Solid Edge part; units mm, degrees
sketch "Sketch1" plane through (0, 0, 0) normal (0, -1, 0) x (1, 0, 0)
  line L0 (-17.399, 15.748) -> (-17.399, -15.748)
  arc A0 (-17.399, -15.748) -> (-15.748, -17.399) centre (-15.748, -15.748) ccw
  line L1 (-15.748, -17.399) -> (15.748, -17.399)
  arc A1 (15.748, -17.399) -> (17.399, -15.748) centre (15.748, -15.748) ccw
  line L2 (17.399, -15.748) -> (17.399, 15.748)
  arc A2 (17.399, 15.748) -> (15.748, 17.399) centre (15.748, 15.748) ccw
  line L3 (15.748, 17.399) -> (-15.748, 17.399)
  arc A3 (-15.748, 17.399) -> (-17.399, 15.748) centre (-15.748, 15.748) ccw
  arc A4 (-19.05, -15.748) -> (-15.748, -19.05) centre (-15.748, -15.748) ccw
  line L4 (-15.748, -19.05) -> (15.748, -19.05)
  arc A5 (15.748, -19.05) -> (19.05, -15.748) centre (15.748, -15.748) ccw
  line L5 (19.05, -15.748) -> (19.05, 15.748)
  arc A6 (19.05, 15.748) -> (15.748, 19.05) centre (15.748, 15.748) ccw
  line L6 (15.748, 19.05) -> (-15.748, 19.05)
  arc A7 (-15.748, 19.05) -> (-19.05, 15.748) centre (-15.748, 15.748) ccw
  line L7 (-19.05, 15.748) -> (-19.05, -15.748)
extrude "Protrusion1" add sketch "Sketch1" against normal blind 44.45
properties material "Steel"
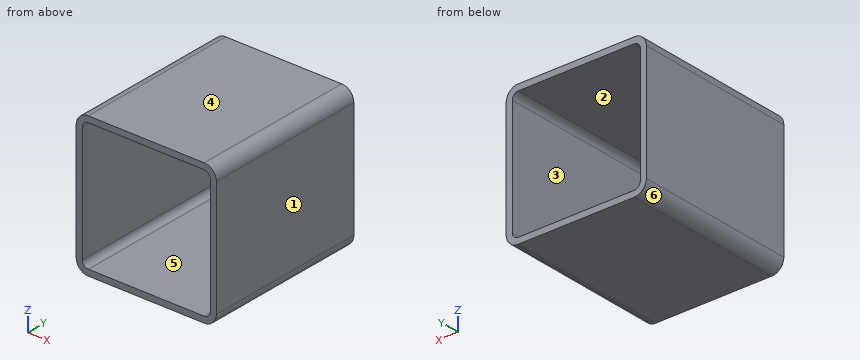
Verification items for the finished model (mm, model axes). Face numbers are marked on the shaded views. A direction names the side the tool comes from. Give positions to 0.01 mm unless a question says otherwise; leave off trailing zeros. Write each loop counter-clockwise with the first axis right and the second up, starting at its lowest first coordinate (ties: lowest second). Pieces come first, ordered by that corner, then holes. Notation, with made-up numbers: M -20,35 L 17,35 A17 cw 17,63 Z; hole C 54.5,47.25 d2. An arc over 180 degrees is marked long. Write item = value, one per line.
(1) Sectioned sample at B-B (x = -1). Record the cut outline in (y, z), then the cut area to 3 significant figures.
Found:
outline = M 0,-19.05 L 44.45,-19.05 L 44.45,-17.4 L 0,-17.4 Z; M 0,17.4 L 44.45,17.4 L 44.45,19.05 L 0,19.05 Z
area = 147 mm2
(2) Access from +Z, -Z, +X, -X, +Y, -Y to the whole of each face (thin tool, end or side, straight path). Record for the marked faces 5 and 6.
Found:
face_5 = +Y, -Y
face_6 = -Z, -X, +Y, -Y
(3) Material ranges on line 1 (X direction, y = 40, z = -5.5); line 2 (X direction, y = 3, z = 17.5), recorded low to high.
Found:
line_1 = -19.05 to -17.4, 17.4 to 19.05
line_2 = -18.55 to 18.55
(4) Draft check along Z on the marked faces 1, 2, 3 and 4. Enter one of: released by +Z, released by -Z, zero draft, split by the parting line, or undercut.
Found:
face_1 = zero draft
face_2 = undercut
face_3 = undercut
face_4 = released by +Z
(5) Sectioned sample at A-A (z = 2). Record the cut outline in (x, y).
Found:
outline = M -19.05,0 L -17.4,0 L -17.4,44.45 L -19.05,44.45 Z; M 17.4,0 L 19.05,0 L 19.05,44.45 L 17.4,44.45 Z
(6) Sectioned sample at C-C (y = 37). Record the cut outline in (x, z).
Found:
outline = M -19.05,-15.75 A3.3 ccw -15.75,-19.05 L 15.75,-19.05 A3.3 ccw 19.05,-15.75 L 19.05,15.75 A3.3 ccw 15.75,19.05 L -15.75,19.05 A3.3 ccw -19.05,15.75 Z; hole M -17.4,-15.75 A1.65 ccw -15.75,-17.4 L 15.75,-17.4 A1.65 ccw 17.4,-15.75 L 17.4,15.75 A1.65 ccw 15.75,17.4 L -15.75,17.4 A1.65 ccw -17.4,15.75 Z
